Part print with two shaded views. Sizes in mm from the minimum x, y, z corner. A direction names the side the tool comes from. Round coordinates to 2 decimals unless told otherwise and drop trailing zeros. Order: outer loops, then holes, each group sorted by start corner. A loop starts at its lowest first (then second) coordinate and runs counter-clockwise, first axis right, second up. Notation, with made-up numbers: (-15.5, 73) -> (-3.5, 73) arc R31 cw to (-3.5, 111) -> close; hole circle Ø1 at (-3, -31). An arc over 180 degrees is marked (long way). Answer as a JSON object with one key per item and string values.
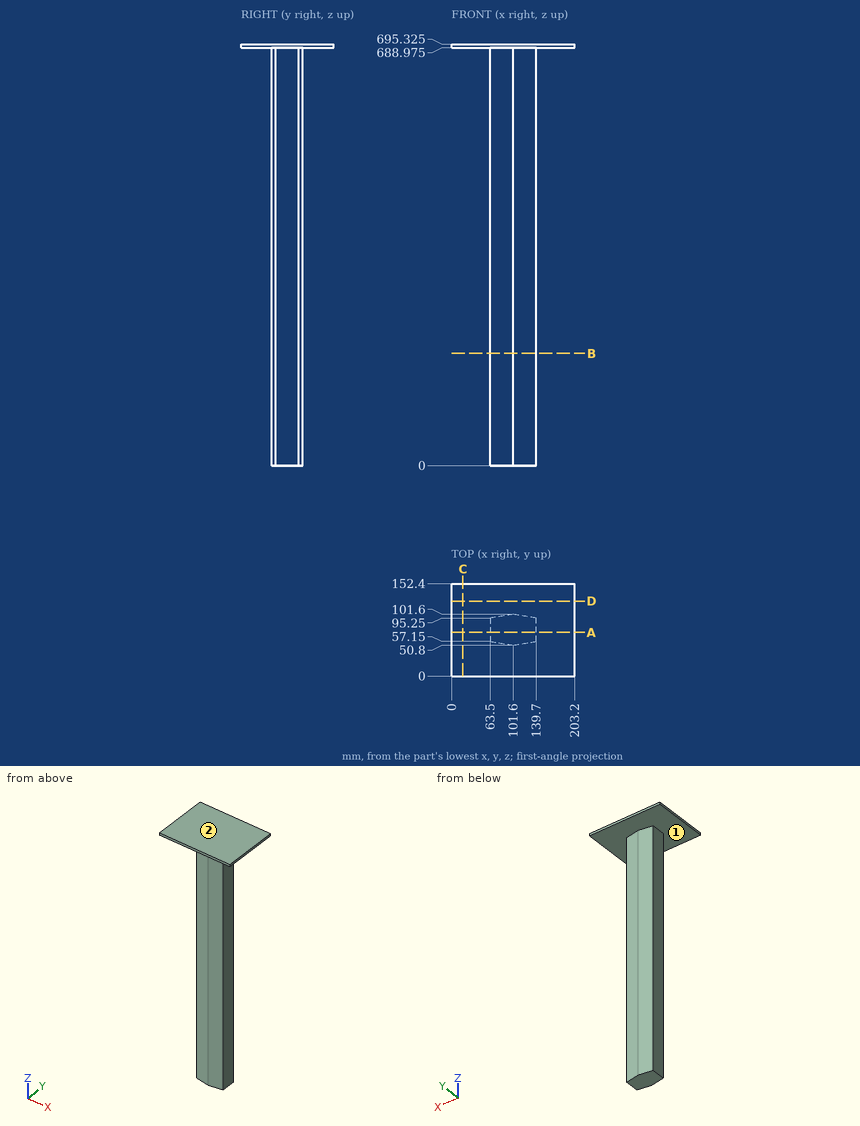
1) Which spindle directions (+Z, -Z, +X, -X, +Y, -Y) get a long thin tool onto all of the face, cutting with end or side? Do the marked faces 1 and 2. Say none if no direction does.
Checked values:
{"face 1": "-Z", "face 2": "+Z, +X, -X, +Y, -Y"}
2) Flat gauge pins, fed straight in: pin 1 Ø10 at (y, z) = (61.5, 281) entering from -X; pin 2 Ø6 at (x, z) = (103.5, 377.5) entering from -Y; pin 3 Ø19 at (y, z) = (72, 512) entering from +X. Where does each tip first touch, or does it go through?
Checked values:
{"pin 1": "stops at x = 63.5", "pin 2": "stops at y = 50.8", "pin 3": "stops at x = 139.7"}
3) Cut at C-C, the plane x = 18.5. Give the cut face in (y, z) (3 decimals).
Checked values:
{"outline": "(0, 688.975) -> (152.4, 688.975) -> (152.4, 695.325) -> (0, 695.325) -> close"}
4) Probe L1, parallel to X at y = 95, z = 119.5; L2, parallel to Z at x = 161, y = 54 (3 decimals); L3, parallel to Y at x = 93, z = 442.5. List the from-to ranges inside material, lowest first. Write a range as from..to.
Checked values:
{"L1": "x = 63.5..139.7", "L2": "z = 688.975..695.325", "L3": "y = 52.23..100.17"}
5) Cut at B-B, the plane z = 185. Give the cut face in (x, y).
Checked values:
{"outline": "(63.5, 57.15) -> (101.6, 50.8) -> (139.7, 57.15) -> (139.7, 95.25) -> (101.6, 101.6) -> (63.5, 95.25) -> close"}
6) Cut at A-A, the plane y = 72. Give the cut face in (x, z) (3 decimals).
Checked values:
{"outline": "(0, 688.975) -> (63.5, 688.975) -> (63.5, 0) -> (139.7, 0) -> (139.7, 688.975) -> (203.2, 688.975) -> (203.2, 695.325) -> (0, 695.325) -> close"}
7) Cut at D-D, the plane y = 123.5. Give the cut face in (x, z) (3 decimals).
Checked values:
{"outline": "(0, 688.975) -> (203.2, 688.975) -> (203.2, 695.325) -> (0, 695.325) -> close"}
